from build123d import *

# Parameters (mm, degrees)
SKETCH4_R           = 8
SKETCH4_W           = 12.4
SKETCH4_H           = 32.25
BOSS_EXTRUDE2_DEPTH = 3


with BuildPart() as part:
    # Sketch4 → Boss-Extrude2 (new body)
    with BuildSketch(Plane(origin=(0, 0, 0), x_dir=(1, 0, 0), z_dir=(0, 1, 0))):
        Polygon((-26, -90), (-9.5, -90), (-9.5, -87), (15.5, -87), (15.5, -90), (32, -90), (32, -78), (29, -78), (29, -56), (32, -56), (32, -34), (29, -34), (29, -12), (32, -12), (32, 0), (15.5, 0), (15.5, -3), (-9.5, -3), (-9.5, 0), (-26, 0), (-26, -12), (-23, -12), (-23, -34), (-26, -34), (-26, -56), (-23, -56), (-23, -78), (-26, -78), align=None)
        with Locations((12.802419237, -37.2)):
            Circle(SKETCH4_R, mode=Mode.SUBTRACT)
        with Locations((-12, -50)):
            Rectangle(SKETCH4_W, SKETCH4_H, mode=Mode.SUBTRACT)
    extrude(amount=BOSS_EXTRUDE2_DEPTH)


solid = part.part
Read the model definition and answer for the solid it produces. Units are mm, in the model's axes. A direction names the side the tool comes from. Round coordinates to 2 decimals unless told otherwise and drop trailing zeros. Write each loop counter-clockwise with the first axis right and the second up, starting at its lowest first coordinate (ties: lowest second). Pieces come first, ordered by that corner, then holes.
Q1. Find section A-A on z = 37.2. Determine the outline of the cut face in (x, y), and give its area (3 significant figures).
Values:
outline: (-26, 0) - (-18.2, 0) - (-18.2, 3) - (-26, 3) - close; (-5.8, 0) - (4.8, 0) - (4.8, 3) - (-5.8, 3) - close; (20.8, 0) - (32, 0) - (32, 3) - (20.8, 3) - close
area: 88.8 mm2
Q2. Find section B-B on z = 64. Determine the outline of the cut face in (x, y), and give its area (3 significant figures).
Values:
outline: (-23, 0) - (-18.2, 0) - (-18.2, 3) - (-23, 3) - close; (-5.8, 0) - (29, 0) - (29, 3) - (-5.8, 3) - close
area: 119 mm2
Q3. Find section D-D on x = 6. Determine the outline of the cut face in (y, z), and give its area (3 significant figures).
Values:
outline: (0, 3) - (3, 3) - (3, 32.99) - (0, 32.99) - close; (0, 41.41) - (3, 41.41) - (3, 87) - (0, 87) - close
area: 227 mm2
Q4. Straight lines are drawn through the part: line 1 (X direction, y = 2.35, z = 37.2); line 2 (X direction, y = 1.65, z = 44.5); line 3 (X direction, y = 0.45, z = 65). For each, find the intervals that lie inside material, in ascending order.
Values:
line 1: x = -26 to -18.2, -5.8 to 4.8, 20.8 to 32
line 2: x = -26 to -18.2, -5.8 to 9.53, 16.08 to 32
line 3: x = -23 to -18.2, -5.8 to 29
Q5. A tool of negligible diameter and unlimited length cuts with its end or side. For faces 5 (the face through (15.5, 1, 1)), 6 (the face through (3, 1, 87)), 7 (the face through (-5.8, 1, 50)), from which of +Z, -Z, +X, -X, +Y, -Y can it reach the whole face along a straight path? Write none if from no direction.
Values:
face 5: -Z, +Y, -Y
face 6: +Z, +Y, -Y
face 7: +Y, -Y
Q6. Find section C-C on y = 1.85. State how many separate pieces and enclosed holes the cut face has, and give its area (3 significant figures).
Values:
separate pieces: 1
enclosed holes: 2
area: 4,210 mm2
Q7. Flat-ended cylindrical pins translate along their axes: P1, Ø1, axis at y = 2.5, z = 57.5, coming from the +X side; P2, Ø4, axis at x = 10.5, z = 48, coming from the -Y side. Find the tip coordinate at first contact, or state that the pin passes through.
Values:
P1: stops at x = 29
P2: stops at y = 0
Q8. The mould has two halves that part along Z. Classify faces 1 (the face through (30, 1, 12)), 2 (the face through (-12, 1, 66.125)), 3 (the face through (32, 1, 45)), 4 (the face through (-18, 1, 90)): released by +Z, released by -Z, zero draft, split by the parting line, or undercut.
Values:
face 1: undercut
face 2: undercut
face 3: zero draft
face 4: released by +Z
